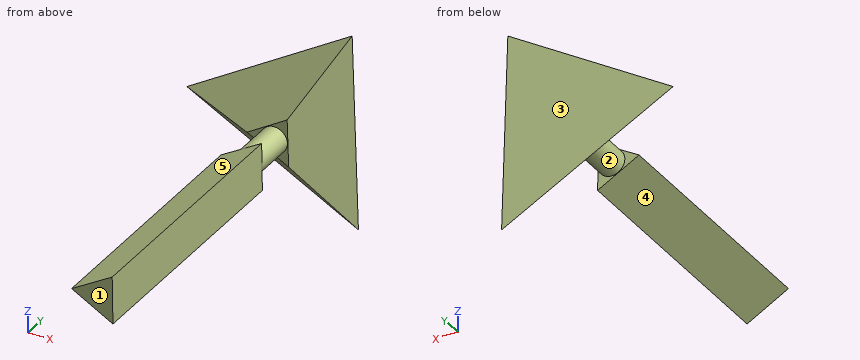
from build123d import *

# Parameters (mm, degrees)
F1_DEPTH = 150
F2_R     = 7.7571961337
F3_DEPTH = 26
F5_DEPTH = 25
F5_TAPER = -45


with BuildPart() as f1:
    # F0 (on Front) → F1 (new body)
    with BuildSketch(Plane.XZ):
        Polygon((7.8226845391, 14.0423364191), (-16.0723623369, -0.2465246729), (8.2496777979, -13.7958117462), align=None)
    extrude(amount=F1_DEPTH)

    # F2 (on Front) → F3 (join)
    with BuildSketch(Plane.XZ):
        Circle(F2_R)
    extrude(amount=-F3_DEPTH)

    # F4 (on face) → F5 (join)
    with BuildSketch(Plane(origin=(0, 26, 0), x_dir=(-1, 0, 0), z_dir=(0, 1, 0))):
        Polygon((-7.5836269453, 14.1686063395), (-8.4785595536, -13.6519167572), (16.0621864989, -0.5166895823), align=None)
    extrude(amount=F5_DEPTH, taper=F5_TAPER)


solid = f1.part
Build history of the part. All positions in model axes, mm. Face numbers are marked on the shaded views. A direction names the side the tool comes from. Give positions to 0.01 mm unless a question says otherwise; leave off trailing zeros. Write each loop counter-clockwise with the first axis right and the second up, starting at its lowest first coordinate (ties: lowest second). Pieces come first, ordered by that corner, then holes. Notation, with made-up numbers: (5, 37.5) - (60, 37.5) arc R16 ccw to (60, 51.5) - close; hole circle Ø2 at (53, -9). An arc over 180 degrees is marked (long way). Use one line per item in the form item = value. Start each with the question number.
1. Band-saw the part on A-A on y = -134.5. Write the cut outline in (x, z), plus the area to 3 significant figures.
2. 3-axis set-ups, long thin cutter, end or side, ignore diameter. For the marked faces 4 and 5: which of +Z, -Z, +X, -X, +Y, -Y reach the whole face in a straight line?
3. Two-plate mould, pull along Y, no slides. Class the marked faces 1, 2 and 3: released by +Y, released by -Y, zero draft, split by the parting line, or undercut.
4. Drop flat-ended pins along their axis: pin 1 Ø1.5 at (x, z) = (-30, 2.5) entering from -Y; pin 2 Ø2 at (y, z) = (-43.5, 13) entering from +X; pin 3 Ø6 at (x, z) = (-45, -9.5) entering from -Y. Give the stop position or say it passes through.
5. Probe line 1 (Y direction, x = -8, z = -28); line 2 (Y direction, x = -33.5, z = 5.5); line 3 (Z direction, x = 2.5, y = 24). List the from-to ranges inside material, lowest first. Write a range as [from, to].
Conclusion:
q1.outline = (-16.07, -0.25) - (8.25, -13.8) - (7.82, 14.04) - close
q1.area = 336 mm²
q2.face_4 = -Z, -X, -Y
q2.face_5 = +Z, -X, -Y
q3.face_1 = released by -Y
q3.face_2 = undercut
q3.face_3 = released by +Y
q4.pin_1 = 35.17
q4.pin_2 = 7.85
q4.pin_3 = 44.58
q5.line_1 = [46.43, 51]
q5.line_2 = [40.31, 51]
q5.line_3 = [-7.34, 7.34]
